Source: CAD feature listing. Evaluate the final solid. Frame: model axes, mm. A direction names the side the tool comes from. Give positions to 0.01 mm unless a question says otherwise; leave off trailing zeros. Loops run counter-clockwise (first coordinate to the right, second up) from the corner with the lowest first, then second, coordinate; pieces in that order, holes last.
```python
from build123d import *

# Parameters (mm, degrees)
SKETCH1_R           = 17.5
SKETCH1_R_2         = 16.5
BOSS_EXTRUDE1_DEPTH = 1.5
SKETCH2_R           = 17.5
BOSS_EXTRUDE2_DEPTH = 5
BOSS_EXTRUDE2_TAPER = 52.4
SKETCH4_R           = 16.5
CUT_EXTRUDE1_DEPTH  = 3
CUT_EXTRUDE1_DRAFT  = -47.3
SKETCH5_R           = 5.5
BOSS_EXTRUDE3_DEPTH = 3
FILLET1_R           = 0.5
SKETCH6_R           = 2
CUT_EXTRUDE2_DEPTH  = 27.509432416
FILLET2_R           = 0.5
FILLET3_R           = 0.5
SKETCH7_R           = 4.25
CUT_EXTRUDE3_DEPTH  = 26.588083301


with BuildPart() as part:
    # Sketch1 → Boss-Extrude1 (new body)
    with BuildSketch(Plane(origin=(0, 0, 0), x_dir=(1, 0, 0), z_dir=(0, 1, 0))):
        with Locations(Location((0, 0, 0), (0, 0, 270))):
            Circle(SKETCH1_R)
        with Locations(Location((0, 0, 0), (0, 0, 270))):
            Circle(SKETCH1_R_2, mode=Mode.SUBTRACT)
    extrude(amount=BOSS_EXTRUDE1_DEPTH)

    # Sketch2 → Boss-Extrude2 (add)
    with BuildSketch(Plane(origin=(0, 1.5, 0), x_dir=(1, 0, 0), z_dir=(0, 1, 0))):
        with Locations(Location((0, 0, 0), (0, 0, 270))):
            Circle(SKETCH2_R)
    extrude(amount=BOSS_EXTRUDE2_DEPTH, taper=BOSS_EXTRUDE2_TAPER)


with BuildPart() as cut_extrude1_tool:
    # Sketch4 → Cut-Extrude1 (with draft: the straight prism first)
    with BuildSketch(Plane.XZ.offset(-1.5)):
        with Locations(Location((0, 0, 0), (0, 0, 270))):
            Circle(SKETCH4_R)
    extrude(amount=-CUT_EXTRUDE1_DEPTH)
    # Cut-Extrude1: the draft: its side faces are tilted about the plane it starts from
    cut_extrude1_sides = [cut_extrude1_tool.faces().sort_by_distance(p)[0] for p in [
        (0, 3, 16.5),
    ]]
    draft(cut_extrude1_sides, Plane.XZ.offset(-1.5), CUT_EXTRUDE1_DRAFT)


with BuildPart() as part_1:
    add(part.part)

    # Cut-Extrude1: cut by cut_extrude1_tool
    add(cut_extrude1_tool.part, mode=Mode.SUBTRACT)

    # Sketch5 → Boss-Extrude3 (add)
    with BuildSketch(Plane(origin=(0, 6.5, 0), x_dir=(1, 0, 0), z_dir=(0, 1, 0))):
        with Locations(Location((0, 0, 0), (0, 0, 270))):
            Circle(SKETCH5_R)
    extrude(amount=BOSS_EXTRUDE3_DEPTH)

    # Fillet1
    fillet1_edges = [part_1.edges().sort_by_distance(p)[0] for p in [
        (0, 9.5, -5.5),
    ]]
    fillet(fillet1_edges, radius=FILLET1_R)

    # Sketch6 → Cut-Extrude2 (cut, through all)
    with BuildSketch(Plane(origin=(0, 9.5, 0), x_dir=(1, 0, 0), z_dir=(0, 1, 0))):
        with Locations(Location((0, 0, 0), (0, 0, 270))):
            Circle(SKETCH6_R)
    extrude(amount=-CUT_EXTRUDE2_DEPTH, mode=Mode.SUBTRACT)

    # Fillet2
    fillet2_edges = [part_1.edges().sort_by_distance(p)[0] for p in [
        (0, 6.5, -5.5),
    ]]
    fillet(fillet2_edges, radius=FILLET2_R)

    # Fillet3
    fillet3_edges = [part_1.edges().sort_by_distance(p)[0] for p in [
        (0, 6.5, -11.007367671),
    ]]
    fillet(fillet3_edges, radius=FILLET3_R)

    # Sketch7 → Cut-Extrude3 (cut, through all)
    with BuildSketch(Plane(origin=(0, 6.5, 0), x_dir=(1, 0, 0), z_dir=(0, 1, 0))):
        with Locations(Location((0, 10.25, 0), (0, 0, 270))):
            Circle(SKETCH7_R)
        with Locations(Location((10.25, 0, 0), (0, 0, 270.673562962))):
            Circle(SKETCH7_R)
        with Locations(Location((0, -10.25, 0), (0, 0, 269.99999999))):
            Circle(SKETCH7_R)
        with Locations(Location((-10.25, 0, 0), (0, 0, 269.326436338))):
            Circle(SKETCH7_R)
    extrude(amount=-CUT_EXTRUDE3_DEPTH, mode=Mode.SUBTRACT)


solid = part_1.part
```
(1) Mould query, pull axis Z, two halves, no side actions, for faces 1 (the conical face through (-10.16, 6.16, 5.28)), 2 (the flat face through (-6, 6.5, 6)), 3 (the conical face through (-5.15, 4.31, -12.43)), 4 (the cylindrical face through (1.277, 5.295, -6.196)). Classes: pulls with the +Z half, pulls with the -Z half, needs draft (parallel to the pull), parting line crosses it, or undercut.
A:
face 1: parting line crosses it
face 2: needs draft
face 3: undercut
face 4: undercut
(2) Section A-A, the plane y = 5. Return the cut outline in (x, z).
A:
outline: (-12.43, -3.65) arc R12.96 ccw to (-3.65, -12.43) arc R4.25 cw (long way) to (3.65, -12.43) arc R12.96 ccw to (12.43, -3.65) arc R4.25 cw (long way) to (12.43, 3.65) arc R12.96 ccw to (3.65, 12.43) arc R4.25 cw (long way) to (-3.65, 12.43) arc R12.96 ccw to (-12.43, 3.65) arc R4.25 cw (long way) to start; hole circle Ø4 at (0, 0)
(3) Reachability of faces 5 (the cylindrical face through (-16.108, 0.74, -3.577)), 6 (the flat face through (-6, 6.5, -6)), 7 (the flat face through (6, 6.5, -6)), 8 (the cylindrical face through (-5.37, 7.99, -1.19)) from +Z, -Z, +X, -X, +Y, -Y: full face, straight path, thin tool, end or side. Return the list, or none.
A:
face 5: -Y
face 6: -Z, -X, +Y
face 7: -Z, +X, +Y
face 8: +Y
(4) First-contact query: pin 1 (5 mm diameter, centred on x = 4, z = 3.5, fed in from +Y); pin 2 (5 mm diameter, centred on x = -5, z = -7, fed in from +Y); pin 3 (5 mm diameter, centred on y = 7, z = 6.5, fed in from -X); pin 4 (3 mm diameter, centred on x = -8.5, y = 4.5, fed in from -Z). Flat tips, straight axial feed; report the tip coordinate or a pass-through.
A:
pin 1: stops at y = 9.5
pin 2: stops at y = 6.5
pin 3: stops at x = -12.16
pin 4: stops at z = -13.21
(5) Ray query, line 1 along X through (y, z) = (5.75, 0); line 2 along X through (y, z) = (2.5, -8); line 3 along Y through (x, z) = (5, 8). Return the intervals inside material, ascending.
A:
line 1: x = -6 to -2, 2 to 6
line 2: x = -14.09 to -13.18, 13.18 to 14.09
line 3: y = 4.5 to 6.5
